Input: part model. Units: mm. Frame: model coordinates. Coordinates: 2 decimals unless noted, no trailing zeros. Write each loop counter-clockwise with the first axis right and the second up, starting at its lowest first coordinate (ties: lowest second). Pieces come first, ordered by that corner, then holes. Notation, with made-up numbers: (57, 20.25) - (98, 20.25) arc R17 ccw to (98, 39.25) - close; hole circle Ø10 at (69, 88). An arc over 180 degrees is marked (long way). Use a Markdown table: item, result. Add a question column.
Q1. Section query C-C (y = -1.2). Give the number of separate pieces and of enclosed holes in the cut face, then the cut area to 3 significant figures.
Q2. Pin query (flat end, axial travel): P1, Ø1.4, axis at y = -1.42, z = 2, coming from the -X side. Return the tip coordinate at first contact, or that it passes through.
Q3. Section query B-B (x = 10). Return the cut outline in (y, z).
Q4. Material intervals for probe 1 along X at (y, z) = (-0.5, 13); probe 2 along Y at (x, z) = (-6.1, 2); probe 3 along Z at (x, y) = (10, -2), sorted ascending. Write a range as from..to.
Q5. Section query A-A (z = 13). Return the cut outline in (x, y).
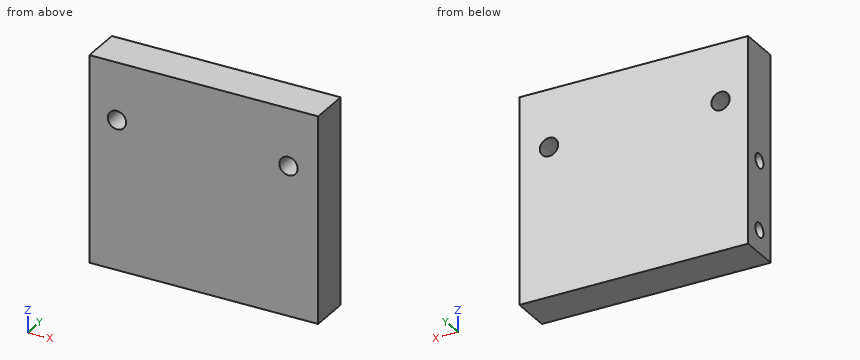
from build123d import *

# Parameters (mm, degrees)
SKETCH_1_W               = 20
SKETCH_1_H               = 3.5
EXTRUDE_1_DEPTH          = 18
SKETCH_2_R               = 0.8
CUT_EXTRUDE_1_DEPTH      = 23.497727458
HOLE_WIZARD_M1_6_1_D     = 1.25
HOLE_WIZARD_M1_6_1_DEPTH = 4
HOLE_WIZARD_M1_6_1_TIP   = 0.375537887


with BuildPart() as part:
    # 草图1 → 凸台-拉伸1 (new body)
    with BuildSketch(Plane.XY):
        with Locations((3.034482759, -1.420060756)):
            Rectangle(SKETCH_1_W, SKETCH_1_H)
    extrude(amount=EXTRUDE_1_DEPTH)

    # 草图2 → 切除-拉伸1 (cut, through all)
    with BuildSketch(Plane(origin=(0, 0.329939244, 0), x_dir=(1, 0, 0), z_dir=(0, 1, 0))):
        with Locations(Location((-4.555517241, -13, 0), (0, 0, 270))):
            Circle(SKETCH_2_R)
        with Locations(Location((10.444482759, -13, 0), (0, 0, 270))):
            Circle(SKETCH_2_R)
    extrude(amount=-CUT_EXTRUDE_1_DEPTH, mode=Mode.SUBTRACT)

    # M1.6 螺纹孔1
    with Locations(Plane.ZY.offset(6.965517241)):
        with Locations((2, -1.420060756), (8, -1.420060756)):
            Hole(HOLE_WIZARD_M1_6_1_D / 2, depth=HOLE_WIZARD_M1_6_1_DEPTH)
            with Locations((0, 0, -(HOLE_WIZARD_M1_6_1_DEPTH + HOLE_WIZARD_M1_6_1_TIP / 2))):  # 118° drill point
                Cone(0, HOLE_WIZARD_M1_6_1_D / 2, HOLE_WIZARD_M1_6_1_TIP, mode=Mode.SUBTRACT)


solid = part.part
Values follow:
| question | item | result |
|---|---|---|
| 1 | separate pieces | 1 |
| 1 | enclosed holes | 2 |
| 1 | area | 346 mm2 |
| 2 | P1 | x = -6.97 |
| 3 | outline | (-3.17, 0) - (0.33, 0) - (0.33, 12.33) - (-3.17, 12.33) - close; (-3.17, 13.67) - (0.33, 13.67) - (0.33, 18) - (-3.17, 18) - close |
| 4 | probe 1 | -6.97..-5.36, -3.76..9.64, 11.24..13.03 |
| 4 | probe 2 | -3.17..-2.05, -0.8..0.33 |
| 4 | probe 3 | 0..12.33, 13.67..18 |
| 5 | outline | (-6.97, -3.17) - (-5.36, -3.17) - (-5.36, 0.33) - (-6.97, 0.33) - close; (-3.76, -3.17) - (9.64, -3.17) - (9.64, 0.33) - (-3.76, 0.33) - close; (11.24, -3.17) - (13.03, -3.17) - (13.03, 0.33) - (11.24, 0.33) - close |
